Check sheet for the modelled part. Datum: model origin and axes. Units: mm. A direction names the side the tool comes from. Round coordinates to 2 decimals unless told otherwise and drop trailing zeros. Write each loop counter-clockwise with the first axis right and the second up, starting at its lowest first coordinate (ties: lowest second). Pieces come first, ordered by that corner, then holes.
Item 1: Release check for a two-part mould opening along Z. For faces 1 (the cylindrical face through (-20.7, 1, -2.4)), 2 (the flat face through (-12.5, 20, 0)), 3 (the flat face through (0, 10, -7.5)) record: pulls with the +Z half, pulls with the -Z half, needs draft (parallel to the pull), parting line crosses it, or undercut.
Item 2: Depth check by flat-ended pin: pin 1 (4 mm diameter, centred on x = 10, z = 4, fed in from +Y); pin 2 (4.5 mm diameter, centred on x = -18, z = -0.5, fed in from -Y); pin 3 (2.5 mm diameter, centred on x = -12.5, y = 7, fed in from +Z); pin 4 (3 mm diameter, centred on x = 17.5, z = -1, fed in from -Y). Enter the tip coordinate at first touch or a pass-through.
Item 3: Material ranges on line 1 along X through (y, z) = (20.5, 0); line 2 along X through (y, z) = (7, -4); line 3 along Z through (x, y) = (-17.5, 15), recorded low to high.
Item 4: Section check A-A, the plane y = 18.5. Record the cut outline in (x, z), plus the area to 3 significant figures.
Item 5: Section check D-D, the plane y = 7. Record the cut outline in (x, z), plus the area to 3 significant figures.
Item 6: Set-up check for faces 4 (the cylindrical face through (-13.852, 8.474, -0.105)), 5 (the flat face through (12.5, 20, 0)), 6 (the cylindrical face through (13.504, 0.986, 0.176)): record each of +Z, -Z, +X, -X, +Y, -Y from which the full face is reachable in a straight line by a thin tool's end or side.
Autodesk Inventor part; units mm, degrees
ref_plane "YZ Plane" through (0, 0, 0) normal (1, 0, 0) x (0, 1, 0)
ref_plane "XZ Plane" through (0, 0, 0) normal (0, 1, 0) x (-1, 0, 0)
ref_plane "XY Plane" through (0, 0, 0) normal (0, 0, 1) x (1, 0, 0)
sketch "Sketch1" plane through (0, 0, 0) normal (0, 0, 1) x (1, 0, 0)
  line L0 (-22.5, 0) -> (22.5, 0)
  line L1 (22.5, 0) -> (22.5, 25)
  line L2 (22.5, 25) -> (12.5, 25)
  line L3 (12.5, 25) -> (12.5, 15)
  line L4 (12.5, 15) -> (-12.5, 15)
  line L5 (-12.5, 15) -> (-12.5, 25)
  line L6 (-12.5, 25) -> (-22.5, 25)
  line L7 (-22.5, 25) -> (-22.5, 0)
  point P0 (0, 0)
  point P1 (0, 0)
  dimension "d0" = 45
  dimension "d1" = 25
  dimension "d2" = 10
  dimension "d3" = 10
extrude "Extrusion1" add sketch "Sketch1" along normal mid plane 15
sketch "Sketch2" plane through (12.5, 25, -7.5) normal (0, 1, 0) x (1, 0, 0)
  line L0 (0, 0) -> (10, 0)
  line L1 (0, 0) -> (0, -15)
  line L2 (10, -15) -> (0, -15)
  line L3 (10, 0) -> (10, -15)
  line L4 (-35, 0) -> (-25, 0)
  line L5 (-35, 0) -> (-35, -15)
  line L6 (-25, -15) -> (-35, -15)
  line L7 (-25, 0) -> (-25, -15)
  line L8 (-25, 0) -> (-25, -15)
  line L9 (5, -7.5) -> (-30, -7.5)
  point P0 (-12.5, -7.5)
  point P1 (-12.5, -7.5)
  dimension "d6" = 35
hole "Hole1" at (17.5, 25, 0) at (-17.5, 25, 0) direction (0, -1, 0) diameter 4 end through all
sketch "Sketch3" plane through (0, 0, 7.5) normal (0, 0, 1) x (1, 0, 0)
  line L0 (12.5, 7) -> (-12.5, 7) construction
  line L1 (0, 0) -> (0, 14) construction
  line L2 (12.5, 15) -> (-12.5, 15)
  point P0 (0, 7)
  dimension "d14" = 8
  dimension "d15" = 25
hole "Hole2" at (12.5, 7, 7.5) at (-12.5, 7, 7.5) direction (0, 0, -1) diameter 4 end through all
sketch "Sketch4" plane through (-22.5, 0, 7.5) normal (0, -1, 0) x (1, 0, 0)
  circle A0 centre (5, -7.5) radius 4
  circle A1 centre (40, -7.5) radius 4
  dimension "d23" = 8
  dimension "d24" = 8
extrude "Extrusion2" cut sketch "Sketch4" against normal blind 4
chamfer "Chamfer1" distance 2 angle 45 2 edges at (-21.5, 4, 0) (13.5, 4, 0)
equation "\"d24\" = d23"
properties part number "sujetador inferior"
Values found:
1. face 1: undercut
1. face 2: needs draft
1. face 3: pulls with the -Z half
2. pin 1: stops at y = 15
2. pin 2: stops at y = 3.04
2. pin 3: passes through
2. pin 4: stops at y = 3.5
3. line 1: x = -22.5 to -19.5, -15.5 to -12.5, 12.5 to 15.5, 19.5 to 22.5
3. line 2: x = -22.5 to -14.5, -10.5 to 10.5, 14.5 to 22.5
3. line 3: z = -7.5 to -2, 2 to 7.5
4. outline: (-22.5, -7.5) - (-12.5, -7.5) - (-12.5, 7.5) - (-22.5, 7.5) - close; (12.5, -7.5) - (22.5, -7.5) - (22.5, 7.5) - (12.5, 7.5) - close; hole circle Ø4 at (-17.5, 0); hole circle Ø4 at (17.5, 0)
4. area: 275 mm2
5. outline: (-22.5, -7.5) - (-14.5, -7.5) - (-14.5, 7.5) - (-22.5, 7.5) - close; (-10.5, -7.5) - (10.5, -7.5) - (10.5, 7.5) - (-10.5, 7.5) - close; (14.5, -7.5) - (22.5, -7.5) - (22.5, 7.5) - (14.5, 7.5) - close; hole circle Ø4 at (-17.5, 0); hole circle Ø4 at (17.5, 0)
5. area: 530 mm2
6. face 4: +Z, -Z
6. face 5: +Z, -Z, +Y
6. face 6: -Y
